Here's the drawing with two shaded views (mm, measured from the low corner). I have some questions. A direction names the side the tool comes from. Give positions to 0.01 mm unless a question says otherwise; leave off trailing zeros. Loops run counter-clockwise (first coordinate to the right, second up) from the corner with the lowest first, then second, coordinate; pieces in that order, holes last. Notation, with made-up numbers: M -26,24 L 32,24 A16 cw 32,44 Z; hole C 26.25,60 d2. An arc over 180 degrees is marked long. Answer in a Markdown table with one row per item. Add a question column.
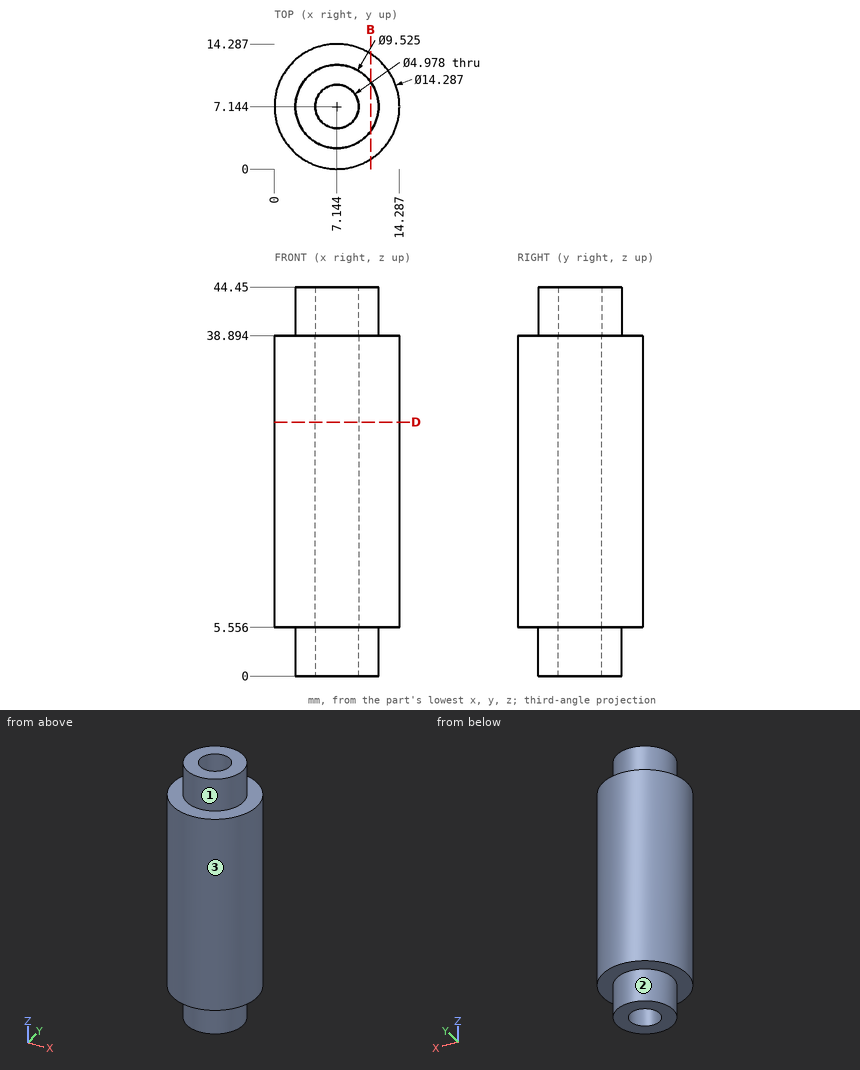
Item 1: Suppose I cut it at D-D (z = 29). List the corners of the cut face in (x, y) for me, then the cut area to 3 significant figures.
Item 2: For the marked faces 1, 2 and 3, which set-ups out of +Z, -Z, +X, -X, +Y, -Y let a thin tool reach every point of the face, with its end or its side?
Item 3: I need wall thicknesses on L1, parallel to X at y = 7, z = 22; L2, parallel to Y at x = 5, z = 20 (1 decimal). Which ranges of each line are inside material? Lowest first, please.
Item 4: Suppose I cut it at B-B (x = 11). List the corners of the cut face in (y, z) for me, then the cut area to 3 significant figures.
Item 5: For P1, Ø2, axis at x = 3, z = 32, coming from the -Y side; P2, Ø4, axis at y = 2.5, z = 29, coming from the -X side; P3, Ø5, axis at y = 12.5, z = 19.5, coming from the +X side, each with a flat end and sliding along its axis, tell me the tip position at first contact or that it passes through.
Values found:
| question | item | result |
|---|---|---|
| 1 | outline | C 7.14,7.14 d14.29; hole C 7.14,7.14 d4.98 |
| 1 | area | 141 mm² |
| 2 | face 1 | +Z |
| 2 | face 2 | -Z |
| 2 | face 3 | +Z, -Z |
| 3 | L1 | 0 to 4.66, 9.63 to 14.29 |
| 3 | L2 | 0.3 to 5.9, 8.4 to 14 |
| 4 | outline | M 1.13,5.56 L 4.35,5.56 L 4.35,0 L 9.94,0 L 9.94,5.56 L 13.16,5.56 L 13.16,38.89 L 9.94,38.89 L 9.94,44.45 L 4.35,44.45 L 4.35,38.89 L 1.13,38.89 Z |
| 4 | area | 463 mm² |
| 5 | P1 | y = 0.73 |
| 5 | P2 | x = 0.51 |
| 5 | P3 | x = 13.69 |
